from build123d import *

# Parameters (mm, degrees)
F0_W     = 970
F0_H     = 545
F0_W_2   = 850
F0_H_2   = 425
F1_DEPTH = 6
F2_R     = 5
F4_D     = 14


with BuildPart() as f1:
    # F0 (on Front) → F1 (new body)
    with BuildSketch(Plane.XZ):
        Rectangle(F0_W, F0_H)
        Rectangle(F0_W_2, F0_H_2, mode=Mode.SUBTRACT)
    extrude(amount=F1_DEPTH)

    # F2
    f2_edges = [f1.edges().sort_by_distance(p)[0] for p in [
        (-485, -3, 272.5),
        (485, -3, 272.5),
        (485, -3, -272.5),
        (-485, -3, -272.5),
    ]]
    fillet(f2_edges, radius=F2_R)

    # F4 (through all)
    with Locations(Plane(origin=(0, 0, 0), x_dir=(1, 0, 0), z_dir=(0, 1, 0))):
        with Locations((462.5, -250), (277.5, -250), (92.5, -250), (-92.5, -250), (-462.5, -250), (-462.5, -150), (-462.5, -50), (-462.5, 50), (-462.5, 150), (-462.5, 250), (-277.5, 250), (-92.5, 250), (92.5, 250), (277.5, 250), (462.5, 250), (462.5, 150), (462.5, 50), (462.5, -50), (462.5, -150), (-277.5, -250)):
            Hole(F4_D / 2)


solid = f1.part
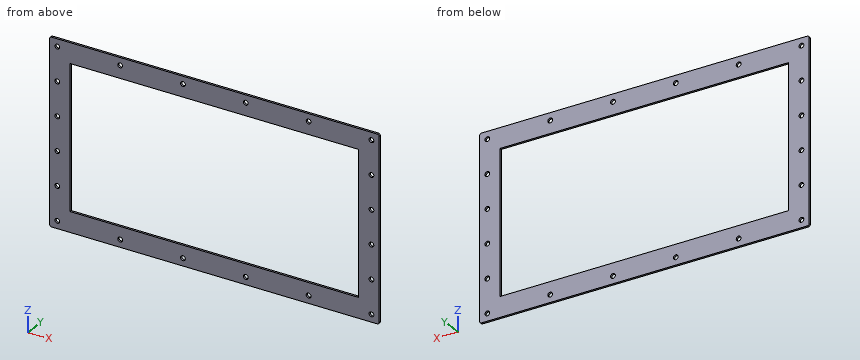
Verification items for the finished model (mm, model axes). Round coordinates to 2 decimals unless told otherwise and drop trailing zeros. Loops run counter-clockwise (first coordinate to the right, second up) from the corner with the lowest first, then second, coordinate; pieces in that order, holes last. Notation, with made-up numbers: (45.25, -2) - (53.25, -2) arc R25 cw to (53.25, 13) - close; hole circle Ø10 at (57.5, 83). An arc over 180 degrees is marked (long way). Use a Markdown table: item, result. Add a question column.
1. Thickness scan on probe 1 along X at (y, z) = (-3.65, 49); probe 2 along X at (y, z) = (-2.2, 50); probe 3 along Z at (x, y) = (211.5, -4.5). Record the ranges inside material, lowest first. Write a range as [from, to].
2. Gauge pin test, flat end, axial feed: pin 1 (8.5 mm diameter, centred on x = 462.5, z = 50, fed in from +Y). Record the tip position at first contact, or that the pin passes through.
3. Section check C-C, the plane y = -1.85. Give the number of separate pieces and of enclosed holes in the cut face, plus the area to 3 significant figures.
4. Section check A-A, the plane x = 403.5. Record the boundary of the cut face in (y, z).
5. Section check B-B, the plane z = 18. Record the boundary of the cut face in (x, y), plus the area to 3 significant figures.
Checks:
| question | item | result |
|---|---|---|
| 1 | probe 1 | x = [-485, -469.43], [-455.57, -425], [425, 455.57], [469.43, 485] |
| 1 | probe 2 | x = [-485, -469.5], [-455.5, -425], [425, 455.5], [469.5, 485] |
| 1 | probe 3 | z = [-272.5, -212.5], [212.5, 272.5] |
| 2 | pin 1 | passes through |
| 3 | separate pieces | 1 |
| 3 | enclosed holes | 21 |
| 3 | area | 164,000 mm^2 |
| 4 | outline | (-6, -272.5) - (0, -272.5) - (0, -212.5) - (-6, -212.5) - close; (-6, 212.5) - (0, 212.5) - (0, 272.5) - (-6, 272.5) - close |
| 5 | outline | (-485, -6) - (-425, -6) - (-425, 0) - (-485, 0) - close; (425, -6) - (485, -6) - (485, 0) - (425, 0) - close |
| 5 | area | 720 mm^2 |
